Part model, mm, in its own coordinate system. Round coordinates to 2 decimals unless told otherwise and drop trailing zeros. Write each loop counter-clockwise with the first axis right and the second up, starting at its lowest first coordinate (ties: lowest second). Pieces come first, ordered by that corner, then holes. Notation, with made-up numbers: (85, -31.75) -> (132, -31.75) arc R25 cw to (132, -10.75) -> close; hole circle Ø4 at (60.5, -4.5). An arc over 180 degrees is marked (long way). Return JSON: item names as keys, results as strings. Group by question number.
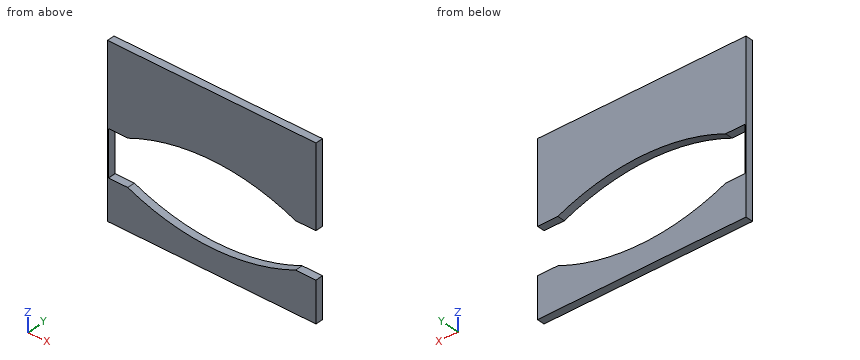
```python
from build123d import *

# Parameters (mm, degrees)
F0_W     = 520.7
F0_H     = 419.1
F1_DEPTH = 19.05
F3_W     = 520.7
F3_H     = 114.3
F4_DEPTH = 25.4
F6_DEPTH = 25.4
F7_W     = 2.54
F7_H     = 243.400686
F8_DEPTH = 19.05


with BuildPart() as f1:
    # F0 (on Front) → F1 (new body)
    with BuildSketch(Plane.XZ):
        Rectangle(F0_W, F0_H)
    extrude(amount=-F1_DEPTH)

    # F3 (on face) → F4 (cut)
    with BuildSketch(Plane.XZ):
        with Locations((0, -50.8)):
            Rectangle(F3_W, F3_H)
    extrude(amount=-F4_DEPTH, mode=Mode.SUBTRACT)

    # F5 (on face) → F6 (cut)
    with BuildSketch(Plane.XZ):
        with BuildLine():
            ThreePointArc((-307.509387, -50.8), (0, -152.4), (307.509387, -50.8))
            ThreePointArc((307.509387, -50.8), (0, 50.8), (-307.509387, -50.8))
        make_face()
    extrude(amount=-F6_DEPTH, mode=Mode.SUBTRACT)

    # F7 (on face) → F8 (join, through all)
    with BuildSketch(Plane.XZ):
        with Locations((-259.08, -28.190974)):
            Rectangle(F7_W, F7_H)
    extrude(amount=-F8_DEPTH)


solid = f1.part
```
Item 1: Cut at C-C (y = 6.5). Write the cut outline in (x, z), then the cut area to 3 significant figures.
Item 2: Cut at B-B (z = -125). Write the cut outline in (x, y), then the cut area to 3 significant figures.
Item 3: Flat gauge pins, fed straight in: P1, Ø12, axis at x = 144.5, z = 137, coming from the -Y side; P2, Ø10, axis at y = 9.5, z = -46, coming from the +X side. Where does each tip first touch, or does it go through?
Item 4: Wall check: L1, parallel to X at y = 16.25, z = -88; L2, parallel to Z at x = -146.5, y = 12.5; L3, parallel to Z at x = -136, y = 12. Give the ranges that are in metal, low to high.
Item 5: Cut at A-A (x = 216). Write the cut outline in (y, z), then the cut area to 3 significant figures.
Checks:
{
 "1": {"outline": "(-260.35, -209.55) -> (260.35, -209.55) -> (260.35, -107.95) -> (209.55, -107.95) arc R516.16 cw to (-209.55, -107.95) -> (-257.81, -107.95) -> (-257.81, 6.35) -> (-209.55, 6.35) arc R516.16 cw to (209.55, 6.35) -> (260.35, 6.35) -> (260.35, 209.55) -> (-260.35, 209.55) -> close", "area": "134,000 mm2"},
 "2": {"outline": "(-260.35, 0) -> (-165.94, 0) -> (-165.94, 19.05) -> (-260.35, 19.05) -> close; (165.94, 0) -> (260.35, 0) -> (260.35, 19.05) -> (165.94, 19.05) -> close", "area": "3,600 mm2"},
 "3": {"P1": "stops at y = 0", "P2": "stops at x = -257.81"},
 "4": {"L1": "x = -260.35 to -257.81", "L2": "z = -209.55 to -131.17, 29.57 to 209.55", "L3": "z = -209.55 to -134.16, 32.56 to 209.55"},
 "5": {"outline": "(0, -209.55) -> (19.05, -209.55) -> (19.05, -107.95) -> (0, -107.95) -> close; (0, 6.35) -> (19.05, 6.35) -> (19.05, 209.55) -> (0, 209.55) -> close", "area": "5,810 mm2"}
}
